```python
from build123d import *

# Parameters (mm, degrees)
SKETCH_1_W          = 16
SKETCH_1_H          = 3.2
SKETCH_1_W_2        = 16.095473014
EXTRUDE_1_DEPTH     = 25
SKETCH_2_R          = 1.5
CUT_EXTRUDE_1_DEPTH = 13.5
SKETCH_3_R          = 1.5
CUT_EXTRUDE_2_DEPTH = 13.5
FILLET_6_R          = 10
FILLET_7_R          = 1.5
CHAMFER_1_SIZE      = 5
FILLET_8_R          = 10
SKETCH1_W           = 21
SKETCH1_H           = 8
CUT_EXTRUDE1_DEPTH  = 7


with BuildPart() as part:
    # Эскиз1 → Бобышка-Вытянуть1 (new body)
    with BuildSketch(Plane(origin=(0, 0, 0), x_dir=(1, 0, 0), z_dir=(0, 1, 0))):
        Polygon((-12.5, -25), (0, -25), (0, -50), (12.5, -50), (12.5, 50), (0, 50), (0, 25), (-12.5, 25), align=None)
        with Locations((-2.5, -16.75)):
            Rectangle(SKETCH_1_W, SKETCH_1_H, mode=Mode.SUBTRACT)
        with Locations((-2.5, 16.75)):
            Rectangle(SKETCH_1_W_2, SKETCH_1_H, mode=Mode.SUBTRACT)
    extrude(amount=EXTRUDE_1_DEPTH)

    # Эскиз2 → Вырез-Вытянуть1 (cut, through all)
    with BuildSketch(Plane.ZY):
        with Locations((-45, 6.5)):
            Circle(SKETCH_2_R)
        with Locations((-45, 18.5)):
            Circle(SKETCH_2_R)
    extrude(amount=-CUT_EXTRUDE_1_DEPTH, mode=Mode.SUBTRACT)

    # Эскиз3 → Вырез-Вытянуть2 (cut, through all)
    with BuildSketch(Plane.ZY):
        with Locations((45, 6.5)):
            Circle(SKETCH_3_R)
        with Locations((45, 18.5)):
            Circle(SKETCH_3_R)
    extrude(amount=-CUT_EXTRUDE_2_DEPTH, mode=Mode.SUBTRACT)

    # Скругление6
    fillet_6_edges = [part.edges().sort_by_distance(p)[0] for p in [
        (-12.5, 12.5, 25),
        (-12.5, 12.5, -25),
    ]]
    fillet(fillet_6_edges, radius=FILLET_6_R)

    # Скругление7
    fillet_7_edges = [part.edges().sort_by_distance(p)[0] for p in [
        (-10.5, 12.5, 15.15),
        (-10.5, 12.5, 18.35),
        (5.5, 12.5, 18.35),
        (5.5, 12.5, 15.15),
        (-10.547736507, 12.5, -18.35),
        (-10.547736507, 12.5, -15.15),
        (5.547736507, 12.5, -15.15),
        (5.547736507, 12.5, -18.35),
    ]]
    fillet(fillet_7_edges, radius=FILLET_7_R)

    # Фаска1
    chamfer_1_edges = [part.edges().sort_by_distance(p)[0] for p in [
        (6.25, 25, 50),
        (6.25, 25, -50),
    ]]
    chamfer(chamfer_1_edges, length=CHAMFER_1_SIZE)

    # Скругление8
    fillet_8_edges = [part.edges().sort_by_distance(p)[0] for p in [
        (0, 12.5, 25),
        (0, 12.5, -25),
    ]]
    fillet(fillet_8_edges, radius=FILLET_8_R)

    # Sketch1 → Cut-Extrude1 (cut)
    with BuildSketch(Plane.XZ):
        with Locations((-2, 16.75)):
            Rectangle(SKETCH1_W, SKETCH1_H)
        with Locations((-2, -16.75)):
            Rectangle(SKETCH1_W, SKETCH1_H)
    extrude(amount=-CUT_EXTRUDE1_DEPTH, mode=Mode.SUBTRACT)


solid = part.part
```
The listing builds one solid part. Answer for the finished solid, in the listing's coordinates (mm). A direction names the side the tool comes from. Give positions to 0.01 mm unless a question says otherwise; leave off trailing zeros. Loops run counter-clockwise (first coordinate to the right, second up) from the corner with the lowest first, then second, coordinate; pieces in that order, holes last. Notation, with made-up numbers: (-17, 1) - (11, 1) arc R27 cw to (11, 18) - close; hole circle Ø11 at (72, 70). An arc over 180 degrees is marked (long way). Answer as CSV lines item,"result". Start each with the question number.
Item 1: The mould has two halves that part along Z. Classify faces 4 (the face through (0, 12, 42)), 5 (the face through (8.5, 3, -17)), 6 (the face through (-10.84, 12.68, -20.52)): +Z half, -Z half, draft (parallel to the pull), parting line (faces both ways), or undercut.
Item 2: A cutting plane is placed at A-A on y = 18.5. Count the separate pieces of the cut face and the enclosed holes in it, then the cut area to 3 significant figures.
Item 3: A cutting plane is placed at C-C on z = 35.5. Determine the outline of the cut face in (x, y).
Item 4: Find the intervals of material crossed by line 1 (Y direction, x = 4.75, z = 45); line 2 (Z direction, x = 5, y = 23.5); line 3 (Z direction, x = -9.5, y = 18.5), in increasing order. Write a range as from..to.
Item 5: For faces 1 (the face through (-2, 3, -12.75)), 2 (the face through (-3, 16, -18.35)), 3 (the face through (6, 10, 50)), determine the directions among +Z, -Z, +X, -X, +Y, -Y from which every point of the face is accessible in a straight line to the end or side of a thin tool.
Item 6: Each of these flat-tipped pins is pushed along its axis until it touches: pin 1 (1.5 mm diameter, centred on x = -2, y = 18, fed in from +Z); pin 2 (4 mm diameter, centred on x = -4, y = 16, fed in from +Z); pin 3 (6.5 mm diameter, centred on x = 2.5, z = -16.5, fed in from -Y). Where does it stop, or does it pass through?
Found:
1,face 4,"draft"
1,face 5,"undercut"
1,face 6,"-Z half"
2,separate pieces,"3"
2,enclosed holes,"2"
2,area,"1,680 mm^2"
3,outline,"(0, 0) - (12.5, 0) - (12.5, 25) - (0, 25) - close"
4,line 1,"y = 0..5, 8..17, 20..25"
4,line 2,"z = -46.5..-18.01, -15.49..15.53, 17.97..46.5"
4,line 3,"z = -22.14..-18.28, -15.22..15.24, 18.26..22.14"
5,face 1,"-X, -Y"
5,face 2,"+Y, -Y"
5,face 3,"+Z, +X, -X, +Y, -Y"
6,pin 1,"stops at z = 28.7"
6,pin 2,"stops at z = 27.54"
6,pin 3,"stops at y = 7"
